```python
from build123d import *

# Parameters (mm, degrees)
ESQUISSE1_W        = 57.14738142
ESQUISSE1_H        = 69.935606632
ESQUISSE1_R        = 1.9
BOSS_EXTRU_7_DEPTH = 1.6
ESQUISSE6_W        = 7.9
ESQUISSE6_H        = 37.7
BOSS_EXTRU_8_DEPTH = 5.34
ESQUISSE7_W        = 56.9
ESQUISSE7_H        = 5.9
BOSS_EXTRU_9_DEPTH = 10.36


with BuildPart() as part:
    # Esquisse1 → Boss.-Extru.7 (new body)
    with BuildSketch(Plane(origin=(0, 0, 0), x_dir=(1, 0, 0), z_dir=(0, 1, 0))):
        with Locations((28.57369071, 34.967803316)):
            Rectangle(ESQUISSE1_W, ESQUISSE1_H)
        with Locations((20.5, 31.935606632)):
            Circle(ESQUISSE1_R, mode=Mode.SUBTRACT)
        with Locations((36.64738142, 31.935606632)):
            Circle(ESQUISSE1_R, mode=Mode.SUBTRACT)
    extrude(amount=BOSS_EXTRU_7_DEPTH)

    # Esquisse6 → Boss.-Extru.8 (add)
    with BuildSketch(Plane(origin=(0, 1.6, 0), x_dir=(1, 0, 0), z_dir=(0, 1, 0))):
        with Locations((53.155892473, 29.734566664)):
            Rectangle(ESQUISSE6_W, ESQUISSE6_H)
        with Locations((4.178526772, 29.710022265)):
            Rectangle(ESQUISSE6_W, ESQUISSE6_H)
    extrude(amount=BOSS_EXTRU_8_DEPTH)

    # Esquisse7 → Boss.-Extru.9 (add)
    with BuildSketch(Plane(origin=(0, 1.6, 0), x_dir=(1, 0, 0), z_dir=(0, 1, 0))):
        with Locations((28.670599558, 52.525606632)):
            Rectangle(ESQUISSE7_W, ESQUISSE7_H)
    extrude(amount=BOSS_EXTRU_9_DEPTH)


solid = part.part
```
Here's how the part is built. I have some questions about the finished solid (model axes, mm). A direction names the side the tool comes from. Coordinates: 2 decimals unless noted, no trailing zeros. Order: outer loops, then holes, each group sorted by start corner. A loop starts at its lowest first (then second) coordinate and runs counter-clockwise, first axis right, second up. Notation, with made-up numbers: (58, 45.25) -> (75, 45.25) arc R35 ccw to (75, 78.25) -> close; hole circle Ø4 at (80, 45.25). An arc over 180 degrees is marked (long way). Return JSON: item names as keys, results as strings.
1) If we section it at B-B on x = 20.5: List the corners of the cut face in (y, z) for me.
Conclusion:
{"outline": "(0, -69.94) -> (1.6, -69.94) -> (1.6, -55.48) -> (11.96, -55.48) -> (11.96, -49.58) -> (1.6, -49.58) -> (1.6, -33.84) -> (0, -33.84) -> close; (0, -30.04) -> (1.6, -30.04) -> (1.6, 0) -> (0, 0) -> close"}
2) If we section it at C-C on z = -47: List the corners of the cut face in (x, y) for me.
Conclusion:
{"outline": "(0, 0) -> (57.15, 0) -> (57.15, 1.6) -> (57.11, 1.6) -> (57.11, 6.94) -> (49.21, 6.94) -> (49.21, 1.6) -> (8.13, 1.6) -> (8.13, 6.94) -> (0.23, 6.94) -> (0.23, 1.6) -> (0, 1.6) -> close"}
3) On a 3-axis mill with a long thin cutter (end or side, diameter ignored), from which of +Z, -Z, +X, -X, +Y, -Y can I reach the whole of each face in a straight line? I mean faces 5 (the flat face through (53, 4, -48.585)), 6 (the cylindrical face through (18.99, 0.79, -30.78)), 7 (the flat face through (4, 6.94, -30)). Say none if no direction works.
Conclusion:
{"face 5": "+X, -X, +Y", "face 6": "+Y, -Y", "face 7": "+Z, +X, -X, +Y"}
4) If we section it at D-D on x = 36: List the corners of the cut face in (y, z) for me.
Conclusion:
{"outline": "(0, -69.94) -> (1.6, -69.94) -> (1.6, -55.48) -> (11.96, -55.48) -> (11.96, -49.58) -> (1.6, -49.58) -> (1.6, -33.72) -> (0, -33.72) -> close; (0, -30.15) -> (1.6, -30.15) -> (1.6, 0) -> (0, 0) -> close"}
5) I'm going to push flat-ended pins straight in: P1, Ø2.5, axis at x = 53.5, y = 4.5, coming from the -Z side; P2, Ø2, axis at y = 5.5, z = -53, coming from the -X side; P3, Ø1.6, axis at y = 5, z = -31.5, coming from the +X side. Where does each tip first touch, or does it pass through?
Conclusion:
{"P1": "stops at z = -55.48", "P2": "stops at x = 0.22", "P3": "stops at x = 57.11"}
6) If I drill on probe 1 along Z at (x, y) = (20.5, 0.65); probe 2 along X at (y, z) = (3.5, -15); probe 3 along Z at (x, y) = (41, 2), over which ranges is the centre line in solid material (lowest first)?
Conclusion:
{"probe 1": "z = -69.94 to -33.84, -30.04 to 0", "probe 2": "x = 0.23 to 8.13, 49.21 to 57.11", "probe 3": "z = -55.48 to -49.58"}
7) If we section it at A-A on y = 3.75: List the corners of the cut face in (x, z) for me.
Conclusion:
{"outline": "(0.22, -55.48) -> (57.12, -55.48) -> (57.12, -49.58) -> (0.22, -49.58) -> close; (0.23, -48.56) -> (8.13, -48.56) -> (8.13, -10.86) -> (0.23, -10.86) -> close; (49.21, -48.58) -> (57.11, -48.58) -> (57.11, -10.88) -> (49.21, -10.88) -> close"}
8) Thinking about a two-plate mould opening in X: for faces 1 (the flat face through (49.206, 4, -29)), 2 (the flat face through (0.229, 4, -29)), 3 (the flat face through (8.129, 4, -29)), 4 (the flat face through (28, 0, -35)), which applies, +X half, -X half, draft (parallel to the pull), parting line (faces both ways), or undercut?
Conclusion:
{"face 1": "undercut", "face 2": "-X half", "face 3": "undercut", "face 4": "draft"}
